Verification items for the finished model (mm, model axes). Face numbers are marked on the shaded views. Round coordinates to 2 decimals unless told otherwise and drop trailing zeros. Loops run counter-clockwise (first coordinate to the right, second up) from the corner with the lowest first, then second, coordinate; pieces in that order, holes last. Notation, with made-up numbers: (88, 13.5) -> (119, 13.5) arc R26 ccw to (119, 31.5) -> close; hole circle Ø1 at (83, 65.5). An arc over 180 degrees is marked (long way). Write item = value, one per line. Start each with the question number.
```python
from build123d import *

# Parameters (mm, degrees)
SKETCH1_W           = 61
SKETCH1_H           = 91
SKETCH1_W_2         = 51
SKETCH1_H_2         = 81
BOSS_EXTRUDE1_DEPTH = 50
SKETCH2_W           = 61
SKETCH2_H           = 91
BOSS_EXTRUDE2_DEPTH = 10
SKETCH3_R           = 5
CUT_EXTRUDE1_DEPTH  = 10


with BuildPart() as part:
    # Sketch1 → Boss-Extrude1 (new body)
    with BuildSketch(Plane.XY):
        Rectangle(SKETCH1_W, SKETCH1_H)
        Rectangle(SKETCH1_W_2, SKETCH1_H_2, mode=Mode.SUBTRACT)
    extrude(amount=BOSS_EXTRUDE1_DEPTH)

    # Sketch2 → Boss-Extrude2 (add)
    with BuildSketch(Plane(origin=(0, 0, 0), x_dir=(-1, 0, 0), z_dir=(0, 0, -1))):
        Rectangle(SKETCH2_W, SKETCH2_H)
    extrude(amount=BOSS_EXTRUDE2_DEPTH)

    # Sketch3 → Cut-Extrude1 (cut)
    with BuildSketch(Plane(origin=(0, 0, -10), x_dir=(-1, 0, 0), z_dir=(0, 0, -1))):
        with Locations((0, -25)):
            Circle(SKETCH3_R)
    extrude(amount=-CUT_EXTRUDE1_DEPTH, mode=Mode.SUBTRACT)


solid = part.part
```
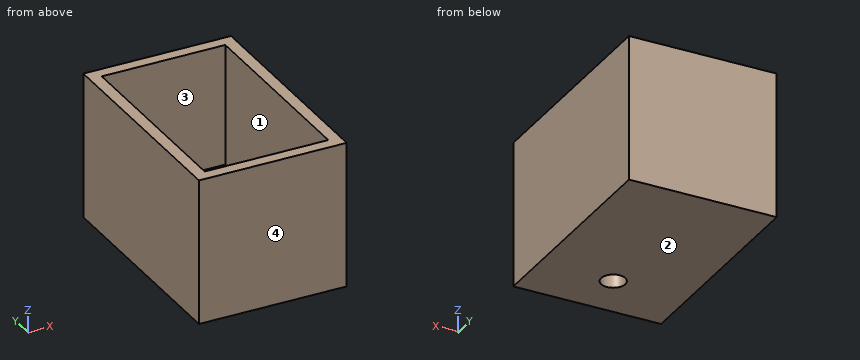
(1) Section check D-D on x = -17. Enter the section's corners in (y, z), then the cut area to 3 significant figures.
(2) Section check C-C on x = 0. Enter the section's corners in (y, z).
(3) Section check B-B on z = 41. Enter the section's corners in (x, y).
(4) Scan lines: line 1 (X direction, y = -24.5, z = 6); line 2 (Y direction, x = -0.5, z = 2.5); line 3 (Y direction, x = 0, z = -4). Record each from-to range of solid material in increasing order. Write a range as [from, to].
(5) Draft check along Y on the marked faces 1, 2, 3 and 4. Enter one of: +Y half, -Y half, draft (parallel to the pull), parting line (faces both ways), or undercut.
(6) Depth check by flat-ended pin: pin 1 Ø5 at (x, y) = (4.5, -28.5) entering from +Z. Enter the tip coordinate at first touch or a pass-through.
(7) Section check A-A on y = -25. Enter the section's corners in (x, z).
Computed values:
q1.outline = (-45.5, -10) -> (45.5, -10) -> (45.5, 50) -> (40.5, 50) -> (40.5, 0) -> (-40.5, 0) -> (-40.5, 50) -> (-45.5, 50) -> close
q1.area = 1,410 mm²
q2.outline = (-45.5, -10) -> (-30, -10) -> (-30, 0) -> (-40.5, 0) -> (-40.5, 50) -> (-45.5, 50) -> close; (-20, -10) -> (45.5, -10) -> (45.5, 50) -> (40.5, 50) -> (40.5, 0) -> (-20, 0) -> close
q3.outline = (-30.5, -45.5) -> (30.5, -45.5) -> (30.5, 45.5) -> (-30.5, 45.5) -> close; hole (-25.5, -40.5) -> (25.5, -40.5) -> (25.5, 40.5) -> (-25.5, 40.5) -> close
q4.line_1 = [-30.5, -25.5], [25.5, 30.5]
q4.line_2 = [-45.5, -40.5], [40.5, 45.5]
q4.line_3 = [-45.5, -30], [-20, 45.5]
q5.face_1 = undercut
q5.face_2 = draft
q5.face_3 = undercut
q5.face_4 = -Y half
q6.pin_1 = 0
q7.outline = (-30.5, -10) -> (-5, -10) -> (-5, 0) -> (-25.5, 0) -> (-25.5, 50) -> (-30.5, 50) -> close; (5, -10) -> (30.5, -10) -> (30.5, 50) -> (25.5, 50) -> (25.5, 0) -> (5, 0) -> close
